Input: dimensioned drawing with shaded views. Units: mm. Origin: part minimum x, y, z. A direction names the side the tool comes from. Round coordinates to 2 decimals unless told otherwise and drop trailing zeros. Loops run counter-clockwise (first coordinate to the right, second up) from the corner with the lowest first, then second, coordinate; pieces in that order, holes last. Notation, with made-up numbers: (32, 35) - (38, 35) arc R33 cw to (38, 74) - close; hole circle Ø5 at (36.5, 55). An arc over 180 degrees is marked (long way). Answer as a JSON object with one key per item and string values. Group by question number.
Item 1: Section C-C (x = 25.75). Return the cut outline in (y, z).
Item 2: Line query: line 1 (Y direction, x = 2.75, z = 1.25); line 2 (X direction, y = 1.5, z = 3.2). Output: solid intervals per line, ascending.
Item 3: Section A-A (z = 2.4). Return the cut outline in (x, y).
Item 4: Reachability of the marked faces 1, 2, 3, 4 and 5 from +Z, -Z, +X, -X, +Y, -Y: full face, straight path, thin tool, end or side. Return the list, or none.
Item 5: Section B-B (y = 27.75). Return the cut outline in (x, z).
Item 6: First-contact query: pin 1 (2 mm diameter, centred on y = 28.5, z = 1.5, fed in from +X); pin 2 (2 mm diameter, centred on y = 2, z = 1.5, fed in from -X); pin 3 (1 mm diameter, centred on x = 21.5, z = 1.5, fed in from +Y). Flat tips, straight axial feed; report the tip coordinate or a pass-through.
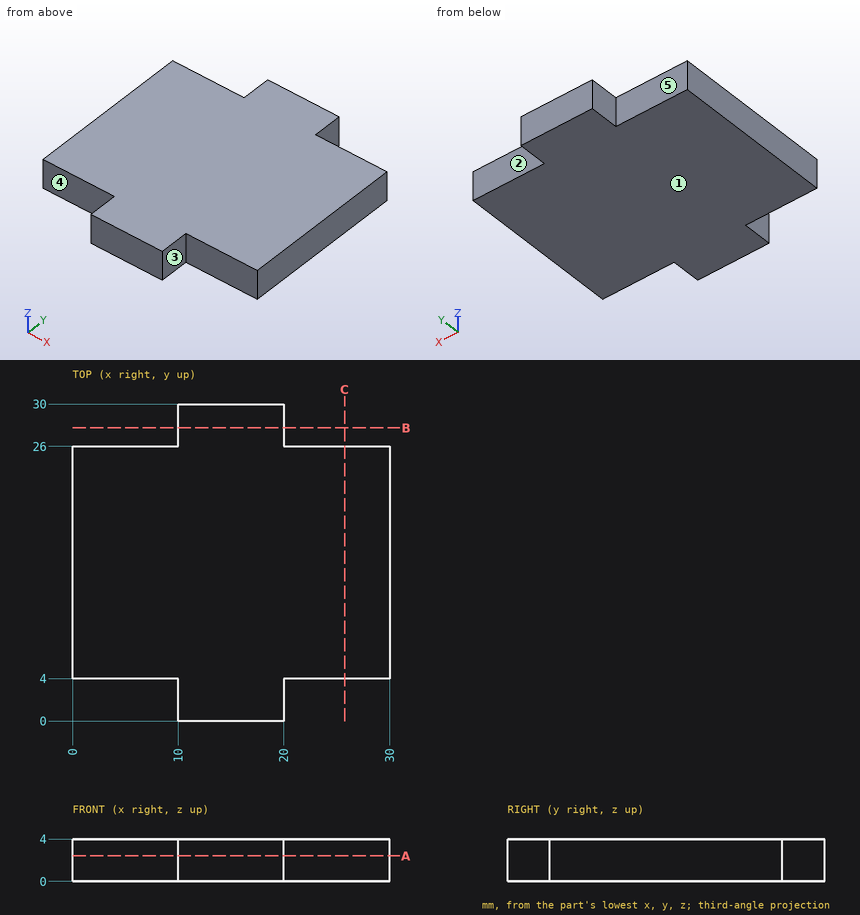
Values:
{
 "1": {"outline": "(4, 0) - (26, 0) - (26, 4) - (4, 4) - close"},
 "2": {"line 1": "y = 4 to 26", "line 2": "x = 10 to 20"},
 "3": {"outline": "(0, 4) - (10, 4) - (10, 0) - (20, 0) - (20, 4) - (30, 4) - (30, 26) - (20, 26) - (20, 30) - (10, 30) - (10, 26) - (0, 26) - close"},
 "4": {"face 1": "-Z, +X, -X, +Y, -Y", "face 2": "+Z, -Z, +X, +Y", "face 3": "+Z, -Z, +X, -Y", "face 4": "+Z, -Z, -X, -Y", "face 5": "+Z, -Z, -X, +Y"},
 "5": {"outline": "(10, 0) - (20, 0) - (20, 4) - (10, 4) - close"},
 "6": {"pin 1": "stops at x = 20", "pin 2": "stops at x = 10", "pin 3": "stops at y = 26"}
}
